from build123d import *

# Parameters (mm, degrees)
EXTRUDE_1_DEPTH     = 20
M10X1_0_1_OUTLINE_R = 4.5
M10X1_0_1_DEPTH     = 86.424893955
FILLET_1_R          = 10
FILLET_2_R          = 20
CHAMFER_1_SIZE      = 10


# Read off the part's stored shape, not the designer's step: M10x1.0 螺纹孔1
with BuildPart() as part:
    # 草图1 → 凸台-拉伸1 (new, symmetric)
    with BuildSketch(Plane(origin=(0, 0, 0), x_dir=(0, 0, -1), z_dir=(1, 0, 0))):
        with BuildLine():
            Line((-235, -105), (165, -105))
            Line((165, -105), (165, -25))
            Line((165, -25), (105, 25))
            Line((105, 25), (85, 25))
            Line((85, 25), (77.5, 0))
            ThreePointArc((77.5, 0), (-26.04083332, -72.994006603), (-60, 49.053542176))
            Line((-60, 49.053542176), (-60, 75))
            Line((-60, 75), (-100, 75))
            Line((-100, 75), (-235, -25))
            Line((-235, -25), (-235, -105))
        make_face()
    extrude(amount=EXTRUDE_1_DEPTH, both=True)

    # M10x1.0 螺纹孔1 outline → M10x1.0 螺纹孔1 (cut)
    with BuildSketch(Plane(origin=(0, 0, 0), x_dir=(1, 0, 0), z_dir=(0, 0.7682212795973757, -0.6401843996644799))):
        with Locations((0, 76.658624366)):
            Circle(M10X1_0_1_OUTLINE_R)
    extrude(amount=M10X1_0_1_DEPTH, mode=Mode.SUBTRACT)

    # 圆角1
    fillet_1_edges = [part.edges().sort_by_distance(p)[0] for p in [
        (0, 75, 60),
        (0, 25, -85),
        (0, 25, -105),
    ]]
    fillet(fillet_1_edges, radius=FILLET_1_R)

    # 圆角2
    fillet_2_edges = [part.edges().sort_by_distance(p)[0] for p in [
        (0, -25, 235),
        (0, 75, 100),
        (0, 49.053542176, 60),
        (0, 0, -77.5),
        (0, -25, -165),
    ]]
    fillet(fillet_2_edges, radius=FILLET_2_R)

    # 倒角1
    chamfer_1_edges = [part.edges().sort_by_distance(p)[0] for p in [
        (-20, -105, 35),
        (20, -105, 35),
    ]]
    chamfer(chamfer_1_edges, length=CHAMFER_1_SIZE)


solid = part.part
Geometry: final body of the model. Coordinates: model frame, mm. A direction names the side the tool comes from. Coordinates: 2 decimals unless noted, no trailing zeros. Order: outer loops, then holes, each group sorted by start corner. A loop starts at its lowest first (then second) coordinate and runs counter-clockwise, first axis right, second up. Notation, with made-up numbers: (-34.75, -26.5) - (-14.75, -26.5) arc R14 ccw to (-14.75, -17.5) - close; hole circle Ø4 at (17, 3). An arc over 180 degrees is marked (long way). Use one line per item in the form item = value.
1) Section C-C (z = 194.5). Return loops of the section in (x, y).
Solutions:
outline = (-20, -95) - (-10, -105) - (10, -105) - (20, -95) - (20, 5) - (-20, 5) - close
2) Section B-B (z = 0). Return loops of the section in (x, y), then the cut area to 3 significant figures.
Solutions:
outline = (-20, -95) - (-10, -105) - (10, -105) - (20, -95) - (20, -77.5) - (-20, -77.5) - close
area = 1,000 mm^2
3) Pin query (flat end, axial travel): pin 1 (3 mm diameter, centred on x = -7, y = 59.5, fed in from -Z); pin 2 (2 mm diameter, centred on x = -4.5, y = -20.5, fed in from +Z); pin 3 (1 mm diameter, centred on x = -7.5, y = -15, fed in from +Z) (3 decimals). Return the tip coordinate at first contact, or that it passes through.
Solutions:
pin_1 = 60
pin_2 = 229.69
pin_3 = 222.175
4) Set-up query: faces 5 (the face through (0.28, 10.37, -80.61)), 6 (the face through (0, -70, -165)), 7 (the face through (0, 25, -97)). Return all of +Z, -Z, +X, -X, +Y, -Y with unobstructed straight access to the full face (end or side cutting, diameter ignored); none if empty.
Solutions:
face_5 = +X, -X, +Y
face_6 = -Z, +X, -X, +Y, -Y
face_7 = -Z, +X, -X, +Y
5) Section A-A (y = -69). Return loops of the section in (x, z), then the cut area to 3 significant figures.
Solutions:
outline = (-20, -165) - (20, -165) - (20, -35.29) - (-20, -35.29) - close; (-20, 35.29) - (20, 35.29) - (20, 235) - (-20, 235) - close
area = 13,200 mm^2
6) Ray query, L1, parallel to Z at x = 9.5, y = -28.5; L2, parallel to Y at x = -7, z = 0; L3, parallel to Z at x = -9, y = 0. Return the intervals inside material, ascending.
Solutions:
L1 = -164.12 to -72.07, 72.07 to 233.89
L2 = -105 to -77.5
L3 = -135 to -77.69, 77.5 to 201.25
7) Mould query, pull axis Y, two halves, no side actions, for faces 1 (the face through (20, -28, 82)), 2 (the face through (0.28, 71.99, 62.85)), 3 (the face through (0.28, -74.17, 22.47)), 4 (the face through (0.28, 49.661, 60.944)). Classes: +Y half, -Y half, draft (parallel to the pull), parting line (faces both ways), or undercut.
Solutions:
face_1 = draft
face_2 = +Y half
face_3 = undercut
face_4 = undercut
